Read the model definition and answer for the solid it produces. Units are mm, in the model's axes. Face numbers are marked on the shaded views. A direction names the side the tool comes from. Coordinates: 2 decimals unless noted, no trailing zeros. Loops run counter-clockwise (first coordinate to the right, second up) from the corner with the lowest first, then second, coordinate; pieces in that order, holes last. Notation, with made-up numbers: (66, -37) -> (95, -37) arc R16 ccw to (95, -16) -> close; hole circle Ø5 at (-3.5, 74). An arc over 180 degrees is marked (long way). Answer in a Markdown table with one row per item.
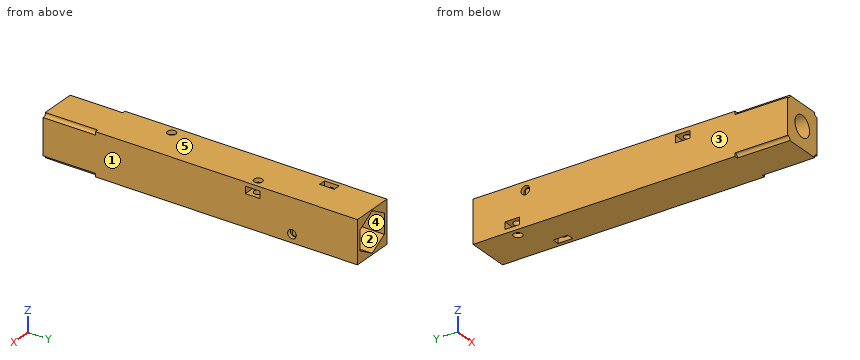
```python
from build123d import *

# Parameters (mm, degrees)
SKETCH_1_W           = 16.2
SKETCH_1_H           = 16.2
SKETCH_1_R           = 4
EXTRUDE_1_DEPTH      = 120
SKETCH_2_R           = 1
CUT_EXTRUDE_1_DEPTH  = 20
CUT_EXTRUDE_2_DEPTH  = 10
SKETCH_4_R           = 1.6
CUT_EXTRUDE_3_DEPTH  = 10
CUT_EXTRUDE_4_DEPTH  = 2.7
SKETCH_6_R           = 1.65
CUT_EXTRUDE_5_DEPTH  = 10
CUT_EXTRUDE_6_DEPTH  = 2.7
SKETCH_9_R           = 1.65
CUT_EXTRUDE_7_DEPTH  = 10
CUT_EXTRUDE_8_DEPTH  = 2.7
SKETCH_11_R          = 1.65
CUT_EXTRUDE_9_DEPTH  = 10
CUT_EXTRUDE_10_DEPTH = 2.7


with BuildPart() as part:
    # Эскиз1 → Бобышка-Вытянуть1 (new body)
    with BuildSketch(Plane(origin=(0, 0, 0), x_dir=(1, 0, 0), z_dir=(0, 1, 0))):
        Rectangle(SKETCH_1_W, SKETCH_1_H)
        with Locations(Location((0, 0, 0), (0, 0, 270))):
            Circle(SKETCH_1_R, mode=Mode.SUBTRACT)
    extrude(amount=EXTRUDE_1_DEPTH)

    # Эскиз2 → Вырез-Вытянуть1 (cut)
    with BuildSketch(Plane.XZ):
        with Locations((-7.8, -7.8)):
            Circle(SKETCH_2_R)
        with Locations((-7.8, 7.8)):
            Circle(SKETCH_2_R)
        with Locations((7.8, 7.8)):
            Circle(SKETCH_2_R)
        with Locations((7.8, -7.8)):
            Circle(SKETCH_2_R)
    extrude(amount=-CUT_EXTRUDE_1_DEPTH, mode=Mode.SUBTRACT)

    # Эскиз3 → Вырез-Вытянуть2 (cut)
    with BuildSketch(Plane(origin=(0, 120, 0), x_dir=(1, 0, 0), z_dir=(0, 1, 0))):
        Polygon((0, 7.621023553), (-6.6, 3.810511777), (-6.6, -3.810511777), (0, -7.621023553), (6.6, -3.810511777), (6.6, 3.810511777), align=None)
    extrude(amount=-CUT_EXTRUDE_2_DEPTH, mode=Mode.SUBTRACT)

    # Эскиз4 → Вырез-Вытянуть3 (cut)
    with BuildSketch(Plane.XY.offset(8.1)):
        with Locations((-5, 40)):
            Circle(SKETCH_4_R)
        with Locations((5, 80)):
            Circle(SKETCH_4_R)
    extrude(amount=-CUT_EXTRUDE_3_DEPTH, mode=Mode.SUBTRACT)

    # Эскиз5 → Вырез-Вытянуть4 (cut)
    with BuildSketch(Plane.XY.offset(6.6)):
        Polygon((-6.616580754, 42.8), (-8.1, 42.8), (-8.1, 37.2), (-6.616580754, 37.2), (-3.383419246, 37.2), (-1.766838493, 40), (-3.383419246, 42.8), align=None)
        Polygon((6.616580754, 82.8), (8.1, 82.8), (8.1, 77.2), (6.616580754, 77.2), (3.383419246, 77.2), (1.766838493, 80), (3.383419246, 82.8), align=None)
    extrude(amount=-CUT_EXTRUDE_4_DEPTH, mode=Mode.SUBTRACT)

    # Эскиз6 → Вырез-Вытянуть5 (cut)
    with BuildSketch(Plane(origin=(0, 0, -8.1), x_dir=(-1, 0, 0), z_dir=(0, 0, -1))):
        with Locations((5, 105)):
            Circle(SKETCH_6_R)
    extrude(amount=-CUT_EXTRUDE_5_DEPTH, mode=Mode.SUBTRACT)

    # Эскиз7 → Вырез-Вытянуть6 (cut)
    with BuildSketch(Plane(origin=(0, 0, -6.6), x_dir=(-1, 0, 0), z_dir=(0, 0, -1))):
        Polygon((6.616580754, 107.8), (8.1, 107.8), (8.1, 102.2), (6.616580754, 102.2), (3.383419246, 102.2), (1.766838493, 105), (3.383419246, 107.8), align=None)
    extrude(amount=-CUT_EXTRUDE_6_DEPTH, mode=Mode.SUBTRACT)

    # Эскиз9 → Вырез-Вытянуть7 (cut)
    with BuildSketch(Plane.ZY.offset(8.1)):
        with Locations((5, 100)):
            Circle(SKETCH_9_R)
    extrude(amount=-CUT_EXTRUDE_7_DEPTH, mode=Mode.SUBTRACT)

    # Эскиз10 → Вырез-Вытянуть8 (cut)
    with BuildSketch(Plane.ZY.offset(6.6)):
        Polygon((6.616580754, 102.8), (8.1, 102.8), (8.1, 97.2), (6.616580754, 97.2), (3.383419246, 97.2), (1.766838493, 100), (3.383419246, 102.8), align=None)
    extrude(amount=-CUT_EXTRUDE_8_DEPTH, mode=Mode.SUBTRACT)

    # Эскиз11 → Вырез-Вытянуть9 (cut)
    with BuildSketch(Plane(origin=(8.1, 0, 0), x_dir=(0, 0, -1), z_dir=(1, 0, 0))):
        with Locations((5, 95)):
            Circle(SKETCH_11_R)
    extrude(amount=-CUT_EXTRUDE_9_DEPTH, mode=Mode.SUBTRACT)

    # Эскиз12 → Вырез-Вытянуть10 (cut)
    with BuildSketch(Plane(origin=(6.6, 0, 0), x_dir=(0, 0, -1), z_dir=(1, 0, 0))):
        Polygon((6.616580754, 97.8), (8.1, 97.8), (8.1, 92.2), (6.616580754, 92.2), (3.383419246, 92.2), (1.766838493, 95), (3.383419246, 97.8), align=None)
    extrude(amount=-CUT_EXTRUDE_10_DEPTH, mode=Mode.SUBTRACT)


solid = part.part
```
1. A tool of negligible diameter and unlimited length cuts with its end or side. For the marked faces 1 and 2, from which of +Z, -Z, +X, -X, +Y, -Y can it reach the whole face along a straight path? Write none if from no direction.
A:
| item | result |
|---|---|
| face 1 | +Z, -Z, +X, +Y, -Y |
| face 2 | +Y |
2. A cutting plane is placed at C-C on z = -5. Give the vertices of the cut face in (x, y).
A:
| item | result |
|---|---|
| outline | (-8.1, 0) -> (8.1, 0) -> (8.1, 93.35) -> (6.6, 93.35) -> (6.6, 92.2) -> (3.9, 92.2) -> (3.9, 93.35) -> (-1.9, 93.35) -> (-1.9, 96.65) -> (3.9, 96.65) -> (3.9, 97.8) -> (6.6, 97.8) -> (6.6, 96.65) -> (8.1, 96.65) -> (8.1, 120) -> (4.54, 120) -> (4.54, 110) -> (-4.54, 110) -> (-4.54, 120) -> (-8.1, 120) -> (-8.1, 107.8) -> (-3.38, 107.8) -> (-1.77, 105) -> (-3.38, 102.2) -> (-8.1, 102.2) -> close |
3. Find the intervals of material crossed by probe 1 along Y at (x, z) = (-0.3, -5); probe 2 along Z at (x, y) = (-0.25, 90); probe 3 along X at (y, z) = (105, -6.95), in increasing order.
A:
| item | result |
|---|---|
| probe 1 | y = 0 to 93.35, 96.65 to 110 |
| probe 2 | z = -8.1 to -3.99, 3.99 to 8.1 |
| probe 3 | x = -8.1 to -6.65, -3.35 to 8.1 |
4. A cutting plane is placed at A-A on y = 88.5. Give the vertices of the cut face in (x, z), and give its area (3 significant figures).
A:
| item | result |
|---|---|
| outline | (-8.1, -8.1) -> (8.1, -8.1) -> (8.1, 8.1) -> (-8.1, 8.1) -> close; hole circle Ø8 at (0, 0) |
| area | 212 mm2 |
5. A cutting plane is placed at D-D on x = 5. Give the vertices of the cut face in (y, z), and give its area (3 significant figures).
A:
| item | result |
|---|---|
| outline | (0, -8.1) -> (92.2, -8.1) -> (92.2, -3.38) -> (95, -1.77) -> (97.8, -3.38) -> (97.8, -8.1) -> (120, -8.1) -> (120, -4.73) -> (110, -4.73) -> (110, 4.73) -> (120, 4.73) -> (120, 8.1) -> (81.6, 8.1) -> (81.6, 6.6) -> (82.8, 6.6) -> (82.8, 3.9) -> (81.6, 3.9) -> (81.6, -1.9) -> (78.4, -1.9) -> (78.4, 3.9) -> (77.2, 3.9) -> (77.2, 6.6) -> (78.4, 6.6) -> (78.4, 8.1) -> (0, 8.1) -> close |
| area | 1,780 mm2 |
6. The mould has two halves that part along Z. Classify the marked faces 3, 4 and 5: pulls with the +Z half, pulls with the -Z half, needs draft (parallel to the pull), parting line crosses it, or undercut.
A:
| item | result |
|---|---|
| face 3 | needs draft |
| face 4 | undercut |
| face 5 | pulls with the +Z half |
7. A cutting plane is placed at B-B on z = 0. Give the vertices of the cut face in (x, y), and give its area (3 significant figures).
A:
| item | result |
|---|---|
| outline | (-8.1, 0) -> (-4, 0) -> (-4, 38.75) arc R1.6 cw (long way) to (-4, 41.25) -> (-4, 103.69) arc R1.65 cw (long way) to (-4, 106.31) -> (-4, 110) -> (-6.6, 110) -> (-6.6, 120) -> (-8.1, 120) -> close; (4, 0) -> (8.1, 0) -> (8.1, 120) -> (6.6, 120) -> (6.6, 110) -> (4, 110) -> (4, 81.25) arc R1.6 cw (long way) to (4, 78.75) -> close |
| area | 911 mm2 |
